Here's how the part is built. I have some questions about the finished solid (model axes, mm). Face numbers are marked on the shaded views. Coordinates: 2 decimals unless noted, no trailing zeros. Loops run counter-clockwise (first coordinate to the right, second up) from the corner with the lowest first, then second, coordinate; pieces in that order, holes last. Notation, with made-up numbers: (-5.5, 77.5) -> (21.5, 77.5) arc R28 ccw to (21.5, 107.5) -> close; hole circle Ø4 at (1.25, 42.5). An arc over 180 degrees is marked (long way). Answer as a JSON object with one key per item and string values. Group by question number.
1) I want a section at B-B (x = 0). Write out the boundary of the cut face in (y, z).
2) I want a section at A-A (z = 0). Write out the boundary of the cut face in (x, y), then the cut area to 3 significant figures.
3) I want a section at C-C (y = -10.25). Write out the boundary of the cut face in (x, z), then the cut area to 3 significant figures.
4) I'm going to push flat-ended pins straight in: pin 1 (3 mm diameter, centred on x = 16, y = -21.5, fed in from -Z); pin 2 (6 mm diameter, centred on y = -12.5, z = 16, fed in from +X); pin 3 (1.5 mm diameter, centred on x = -27.5, y = -22, fed in from -Z). Where does each tip first touch, or does it pass through?
5) If we mould it in two halves opening along Z, with no side actions, what happens to the marked faces 1, 2 and 3? For each: +Z half, -Z half, draft (parallel to the pull), parting line (faces both ways), or undercut.
6) I need wall thicknesses on probe 1 along Z at (x, y) = (0, -8); probe 2 along Z at (x, y) = (-4, -15.75); probe 3 along X at (y, z) = (-14.5, 33). Which ranges of each line are inside material? Lowest first, please. Write a range as [from, to].
```python
from build123d import *

# Parameters (mm, degrees)
F0_R     = 74.258017
F1_DEPTH = 25.4
F2_R     = 44.71295
F3_DEPTH = 25.4
F4_R     = 5.08


with BuildPart() as f1:
    # F0 (on Front) → F1 (new body)
    with BuildSketch(Plane.XZ):
        Circle(F0_R)
    extrude(amount=F1_DEPTH)

    # F2 (on face) → F3 (cut)
    with BuildSketch(Plane.XZ.offset(25.4)):
        Circle(F2_R)
    extrude(amount=-F3_DEPTH, mode=Mode.SUBTRACT)

    # F4
    f4_edges = [f1.edges().sort_by_distance(p)[0] for p in [
        (-74.258017, -25.4, 0),
        (-74.258017, 0, 0),
    ]]
    fillet(f4_edges, radius=F4_R)


solid = f1.part
```
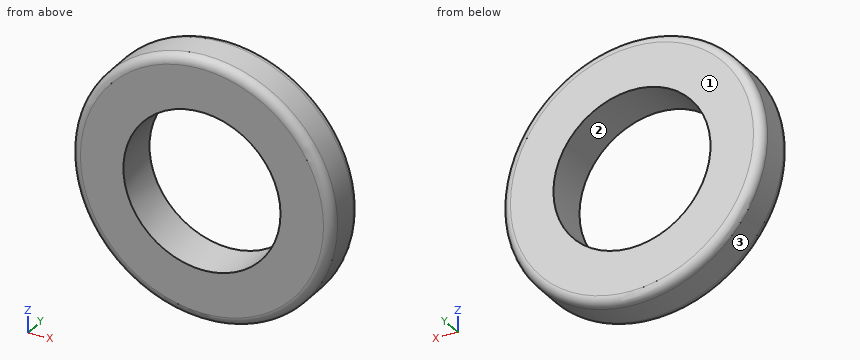
Determined:
{
 "1": {"outline": "(-25.4, -69.18) arc R5.08 ccw to (-20.32, -74.26) -> (-5.08, -74.26) arc R5.08 ccw to (0, -69.18) -> (0, -44.71) -> (-25.4, -44.71) -> close; (-25.4, 44.71) -> (0, 44.71) -> (0, 69.18) arc R5.08 ccw to (-5.08, 74.26) -> (-20.32, 74.26) arc R5.08 ccw to (-25.4, 69.18) -> close"},
 "2": {"outline": "(-74.26, -20.32) arc R5.08 ccw to (-69.18, -25.4) -> (-44.71, -25.4) -> (-44.71, 0) -> (-69.18, 0) arc R5.08 ccw to (-74.26, -5.08) -> close; (44.71, -25.4) -> (69.18, -25.4) arc R5.08 ccw to (74.26, -20.32) -> (74.26, -5.08) arc R5.08 ccw to (69.18, 0) -> (44.71, 0) -> close", "area": "1,480 mm^2"},
 "3": {"outline": "circle Ø148.52 at (0, 0); hole circle Ø89.43 at (0, 0)", "area": "11,000 mm^2"},
 "4": {"pin 1": "z = -72.77", "pin 2": "x = 73.11", "pin 3": "z = -69.05"},
 "5": {"face 1": "draft", "face 2": "undercut", "face 3": "parting line"},
 "6": {"probe 1": "[-74.26, -44.71], [44.71, 74.26]", "probe 2": "[-74.15, -44.53], [44.53, 74.15]", "probe 3": "[-66.52, -30.17], [30.17, 66.52]"}
}
